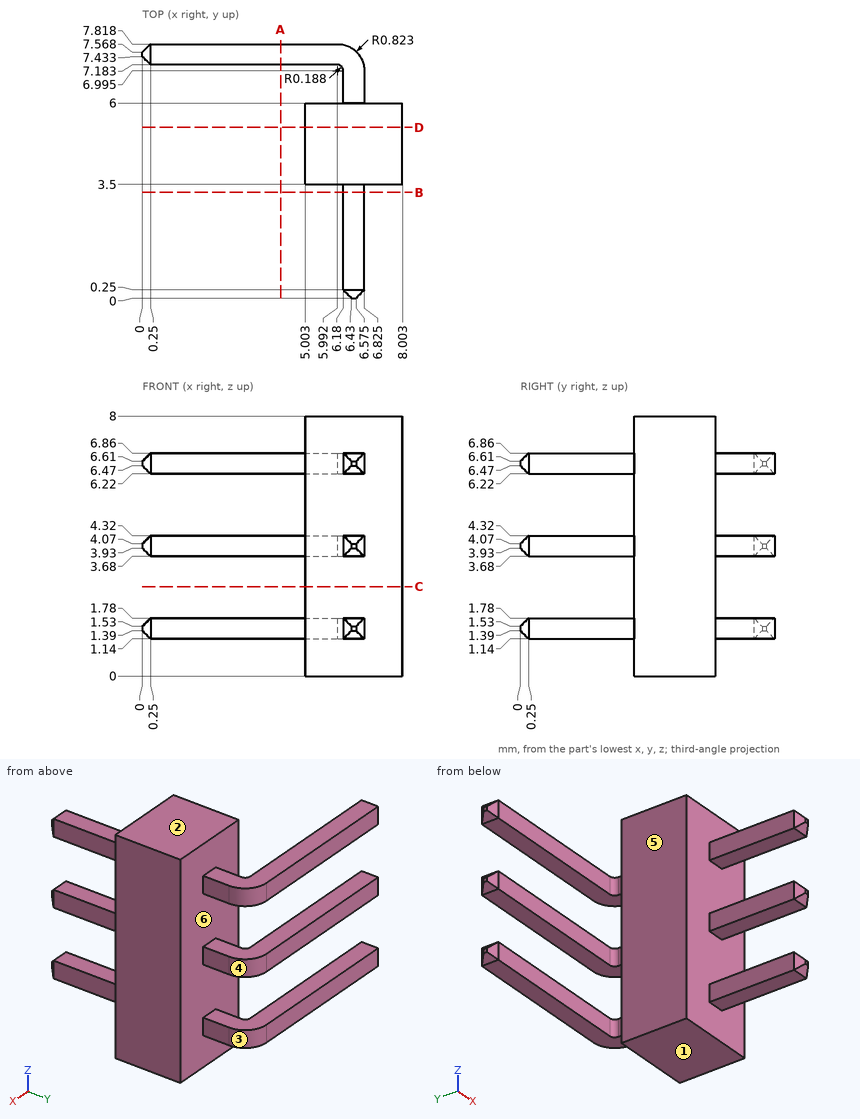
The drawing under review shows one solid part. Ordinate dimensions are in mm from its lowest x, y, z. A direction names the side the tool comes from. Round coordinates to 2 decimals unless told otherwise and drop trailing zeros. Write each loop counter-clockwise with the first axis right and the second up, starting at its lowest first coordinate (ties: lowest second). Pieces come first, ordered by that corner, then holes. Notation, with made-up numbers: (-27.5, 73.25) -> (7.5, 73.25) arc R19 cw to (7.5, 102.25) -> close; hole circle Ø1 at (39, 28). An arc over 180 degrees is marked (long way). One line per question, with ' | ' between items. Start each with the question number.
(1) Tool access review of the marked faces 4, 5 and 6: name each direction out of +Z, -Z, +X, -X, +Y, -Y from which nothing blocks a thin tool from reaching the whole face with its end or side.
(2) For line 1 along Z through (x, y) = (4, 7.5); line 2 along X through (y, z) = (5.25, 3.75); line 3 along Y through (x, z) = (5.25, 6.5), list the stretches that pass through material, from the lowest coordinate up. Write a range as from..to.
(3) Add section C-C, the plane z = 2.75. Write out the cut boundary in (x, y).
(4) Mouldability with a two-part tool opening along Z and no side actions: class the marked faces 1, 2 and 3 as released by +Z, released by -Z, zero draft, split by the parting line, or undercut.
(5) Add section B-B, the plane y = 3.25. Write out the cut boundary in (x, z) (1 decimal).
(6) Insertion check: P1, Ø0.5, axis at y = 6.5, z = 6.5, coming from the +X side (1 decimal); P2, Ø2, axis at x = 3, y = 6.5, coming from the -Z side; P3, Ø0.5, axis at x = 6.5, y = 2, coming from the +Z side. Each pin has a flat end and moves straight along its axis. Give the tip position at first contact, or say it passes through.
(7) Add section A-A, the plane x = 4.25. Write out the cut boundary in (y, z).
(8) Add section D-D, the plane y = 5.25. Write out the cut boundary in (x, z).
Answer list:
1) face 4: +Z, -Z, +X, +Y | face 5: +Z, -Z, -X, -Y | face 6: none
2) line 1: 1.14..1.78, 3.68..4.32, 6.22..6.86 | line 2: 5..8 | line 3: 3.5..6, 7.18..7.82
3) outline: (5, 3.5) -> (8, 3.5) -> (8, 6) -> (5, 6) -> close
4) face 1: released by -Z | face 2: released by +Z | face 3: zero draft
5) outline: (6.2, 1.1) -> (6.8, 1.1) -> (6.8, 1.8) -> (6.2, 1.8) -> close; (6.2, 3.7) -> (6.8, 3.7) -> (6.8, 4.3) -> (6.2, 4.3) -> close; (6.2, 6.2) -> (6.8, 6.2) -> (6.8, 6.9) -> (6.2, 6.9) -> close
6) P1: x = 6.8 | P2: z = 1.14 | P3: z = 6.86
7) outline: (7.18, 1.14) -> (7.82, 1.14) -> (7.82, 1.78) -> (7.18, 1.78) -> close; (7.18, 3.68) -> (7.82, 3.68) -> (7.82, 4.32) -> (7.18, 4.32) -> close; (7.18, 6.22) -> (7.82, 6.22) -> (7.82, 6.86) -> (7.18, 6.86) -> close
8) outline: (5, 0) -> (8, 0) -> (8, 8) -> (5, 8) -> close
